Build history of the part. All positions in model axes, mm. Face numbers are marked on the shaded views. A direction names the side the tool comes from. Coordinates: 2 decimals unless noted, no trailing zeros. Write each loop counter-clockwise with the first axis right and the second up, starting at its lowest first coordinate (ties: lowest second). Pieces come first, ordered by that corner, then holes. Notation, with made-up numbers: M -20.75,-24 L 30.25,-24 A29 cw 30.25,14 Z; hole C 5,61.5 d7. An arc over 180 degrees is marked long. Use CSV: the item, a comma, the result in double quotes. Start each with the question number.
```python
from build123d import *

# Parameters (mm, degrees)
SKETCH2_W           = 42
SKETCH2_H           = 16
BOSS_EXTRUDE1_DEPTH = 4
SKETCH9_W           = 8
SKETCH9_H           = 12
BOSS_EXTRUDE3_DEPTH = 12.2
SKETCH10_W          = 5
SKETCH10_H          = 10
CUT_EXTRUDE6_DEPTH  = 11.7
SKETCH12_R          = 3
CUT_EXTRUDE7_DEPTH  = 8
SKETCH17_W          = 42
SKETCH17_H          = 4
BOSS_EXTRUDE4_DEPTH = 4
SKETCH21_W          = 20
SKETCH21_H          = 4
CUT_EXTRUDE8_DEPTH  = 11
SKETCH22_W          = 20
SKETCH22_H          = 4
CUT_EXTRUDE9_DEPTH  = 11


with BuildPart() as part:
    # Sketch2 → Boss-Extrude1 (new body)
    with BuildSketch(Plane(origin=(0, 0, 0), x_dir=(1, 0, 0), z_dir=(0, 1, 0))):
        with Locations((-19.403711124, -12.332190114)):
            Rectangle(SKETCH2_W, SKETCH2_H)
    extrude(amount=BOSS_EXTRUDE1_DEPTH)

    # Sketch9 → Boss-Extrude3 (add)
    with BuildSketch(Plane(origin=(0, 4, 0), x_dir=(1, 0, 0), z_dir=(0, 1, 0))):
        with Locations((-19.403711124, -14.332190114)):
            Rectangle(SKETCH9_W, SKETCH9_H)
    extrude(amount=BOSS_EXTRUDE3_DEPTH)

    # Sketch10 → Cut-Extrude6 (cut)
    with BuildSketch(Plane(origin=(0, 16.2, 0), x_dir=(1, 0, 0), z_dir=(0, 1, 0))):
        with Locations((-19.403711124, -14.332190114)):
            Rectangle(SKETCH10_W, SKETCH10_H)
    extrude(amount=-CUT_EXTRUDE6_DEPTH, mode=Mode.SUBTRACT)

    # Sketch12 → Cut-Extrude7 (cut)
    with BuildSketch(Plane(origin=(-15.403711124, 0, 0), x_dir=(0, 0, -1), z_dir=(1, 0, 0))):
        with Locations((-14.332190114, 10.1)):
            Circle(SKETCH12_R)
    extrude(amount=-CUT_EXTRUDE7_DEPTH, mode=Mode.SUBTRACT)

    # Sketch17 → Boss-Extrude4 (add)
    with BuildSketch(Plane.XY.offset(20.332190114)):
        with Locations((-19.403711124, 2)):
            Rectangle(SKETCH17_W, SKETCH17_H)
    extrude(amount=BOSS_EXTRUDE4_DEPTH)

    # Sketch21 → Cut-Extrude8 (cut)
    with BuildSketch(Plane.ZY.offset(40.403711124)):
        with Locations((14.332190114, 2)):
            Rectangle(SKETCH21_W, SKETCH21_H)
    extrude(amount=-CUT_EXTRUDE8_DEPTH, mode=Mode.SUBTRACT)

    # Sketch22 → Cut-Extrude9 (cut)
    with BuildSketch(Plane(origin=(1.596288876, 0, 0), x_dir=(0, 0, -1), z_dir=(1, 0, 0))):
        with Locations((-14.332190114, 2)):
            Rectangle(SKETCH22_W, SKETCH22_H)
    extrude(amount=-CUT_EXTRUDE9_DEPTH, mode=Mode.SUBTRACT)


solid = part.part
```
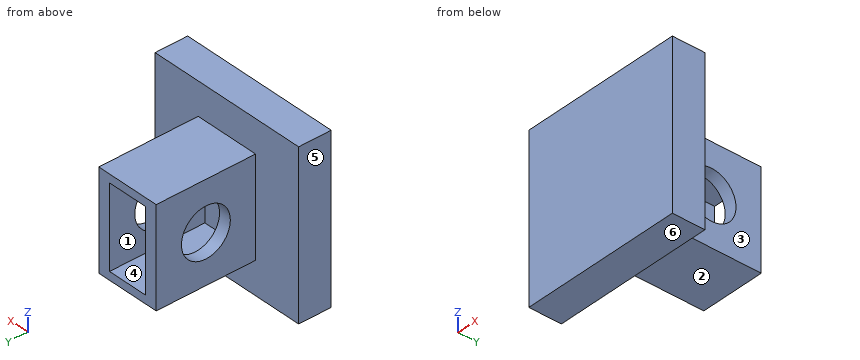
1. Slice it at A-A (y = 10.1). List the corners of the cut face in (x, z).
2. Drill centre lines: line 1 along X through (y, z) = (10.75, 11.25); line 2 along Y through (x, z) = (-21, 21); line 3 along Z through (x, y) = (-20.75, 5.25). Where is each one in solid material? Low to high. Write a range as from..to.
3. Pull direction X, two halves, no side cores. Call the marked faces 4, 5 and 6: pulls with the +X half, pulls with the -X half, needs draft (parallel to the pull), parting line crosses it, or undercut.
4. Slice it at B-B (y = 14.75). List the corners of the cut face in (x, z), and give its area (3 significant figures).
5. Slice it at C-C (x = -17.25). List the corners of the cut face in (y, z), and give its area (3 significant figures).
6. 3-axis set-ups, long thin cutter, end or side, ignore diameter. For the marked faces 1, 2 and 3: which of +Z, -Z, +X, -X, +Y, -Y reach the whole face in a straight line?
7. Slice it at D-D (z = 8.75). List the corners of the cut face in (x, y).
8. Flat gauge pins, fed straight in: pin 1 (1 mm diameter, centred on x = -21, y = 10.5, fed in from +Z); pin 2 (1 mm diameter, centred on y = 8, z = 12.5, fed in from -X); pin 3 (1.5 mm diameter, centred on x = -12, z = 20.5, fed in from +Y). Where does each tip first touch, or does it go through?
Established:
1,outline,"M -23.4,8.33 L -15.4,8.33 L -15.4,11.33 L -16.9,11.33 L -16.9,9.33 L -21.9,9.33 L -21.9,11.33 L -23.4,11.33 Z; M -23.4,17.33 L -21.9,17.33 L -21.9,19.33 L -16.9,19.33 L -16.9,17.33 L -15.4,17.33 L -15.4,20.33 L -23.4,20.33 Z"
2,line 1,"x = -23.4..-21.9, -16.9..-15.4"
2,line 2,"y = 0..4"
2,line 3,"z = 8.33..9.33, 19.33..20.33"
3,face 4,"undercut"
3,face 5,"pulls with the -X half"
3,face 6,"needs draft"
4,outline,"M -23.4,8.33 L -15.4,8.33 L -15.4,20.33 L -23.4,20.33 Z; hole M -21.9,9.33 L -16.9,9.33 L -16.9,19.33 L -21.9,19.33 Z"
4,area,"46.0 mm2"
5,outline,"M 0,4.33 L 4,4.33 L 4,8.33 L 16.2,8.33 L 16.2,9.33 L 4.5,9.33 L 4.5,19.33 L 16.2,19.33 L 16.2,20.33 L 4,20.33 L 4,24.33 L 0,24.33 Z"
5,area,"109 mm2"
6,face 1,"+Y"
6,face 2,"-Z, +X, -X, +Y"
6,face 3,"+Z, -Z, +X, +Y"
7,outline,"M -29.4,0 L -9.4,0 L -9.4,4 L -15.4,4 L -15.4,16.2 L -23.4,16.2 L -23.4,4 L -29.4,4 Z"
8,pin 1,"stops at z = 20.33"
8,pin 2,"stops at x = -23.4"
8,pin 3,"stops at y = 4"
